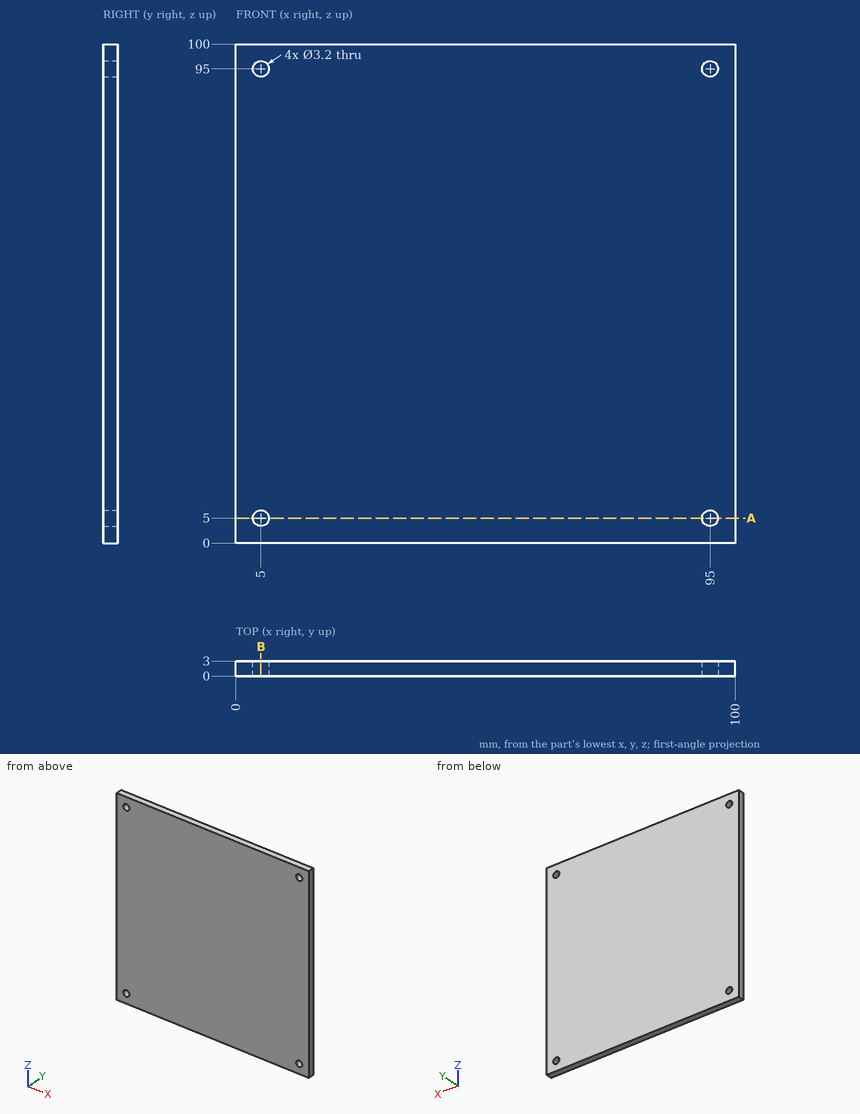
Could you check a few things on this drawing? It's one solid part, dimensions in mm from its lowest x, y, z. Give positions to 0.01 mm unless a question says otherwise; leave off trailing zeros. Write each loop counter-clockwise with the first axis right and the second up, starting at its lowest first coordinate (ties: lowest second). Pieces come first, ordered by that corner, then holes. Notation, with made-up numbers: (63, 53.5) -> (77, 53.5) arc R20 cw to (77, 88.5) -> close; hole circle Ø5 at (-13, 32.5). An arc over 180 degrees is marked (long way). Write each question's results on one line, items separated by ' | '.
1. I want a section at A-A, the plane z = 5. Write out the boundary of the cut face in (x, y), then the cut area to 3 significant figures.
Check sheet entries:
outline: (0, 0) -> (3.4, 0) -> (3.4, 3) -> (0, 3) -> close; (6.6, 0) -> (93.4, 0) -> (93.4, 3) -> (6.6, 3) -> close; (96.6, 0) -> (100, 0) -> (100, 3) -> (96.6, 3) -> close | area: 281 mm²
2. I need wall thicknesses on L1, parallel to X at y = 1.1, z = 95. Which ranges of the line are inside material? Lowest first, please.
Check sheet entries:
L1: x = 0 to 3.4, 6.6 to 93.4, 96.6 to 100
3. I want a section at B-B, the plane x = 5. Write out the boundary of the cut face in (y, z), then the cut area to 3 significant figures.
Check sheet entries:
outline: (0, 0) -> (3, 0) -> (3, 3.4) -> (0, 3.4) -> close; (0, 6.6) -> (3, 6.6) -> (3, 93.4) -> (0, 93.4) -> close; (0, 96.6) -> (3, 96.6) -> (3, 100) -> (0, 100) -> close | area: 281 mm²
